Verification items for the finished model (mm, model axes). Face numbers are marked on the shaded views. A direction names the side the tool comes from. Coordinates: 2 decimals unless noted, no trailing zeros. Loops run counter-clockwise (first coordinate to the right, second up) from the corner with the lowest first, then second, coordinate; pieces in that order, holes last. Notation, with made-up numbers: M 10,-28.5 L 14,-28.5 A20 cw 14,-0.5 Z; hole C -13.5,82 d1. An arc over 180 degrees is marked long. Write item = value, one per line. Start each with the question number.
```python
from build123d import *

# Parameters (mm, degrees)
SKETCH1_W           = 40
SKETCH1_H           = 20
BOSS_EXTRUDE1_DEPTH = 37
BOSS_EXTRUDE2_DEPTH = 2
SKETCH3_R           = 6
BOSS_EXTRUDE3_DEPTH = 2
SKETCH4_R           = 2.75
BOSS_EXTRUDE4_DEPTH = 5
SKETCH5_W           = 7
SKETCH5_H           = 20
BOSS_EXTRUDE5_DEPTH = 3
SKETCH7_R           = 1.75
CUT_EXTRUDE3_DEPTH  = 44.0464865


with BuildPart() as part:
    # Sketch1 → Boss-Extrude1 (new body)
    with BuildSketch(Plane.XY):
        Rectangle(SKETCH1_W, SKETCH1_H)
    extrude(amount=BOSS_EXTRUDE1_DEPTH)

    # Sketch2 → Boss-Extrude2 (add)
    with BuildSketch(Plane.XY.offset(37)):
        with BuildLine():
            Line((-7.5, 10), (20, 10))
            Line((20, 10), (20, -10))
            Line((20, -10), (-7.5, -10))
            ThreePointArc((-7.5, -10), (-17.5, 0), (-7.5, 10))
        make_face()
    extrude(amount=BOSS_EXTRUDE2_DEPTH)

    # Sketch3 → Boss-Extrude3 (add)
    with BuildSketch(Plane.XY.offset(39)):
        with Locations((-7.5, 0)):
            Circle(SKETCH3_R)
    extrude(amount=BOSS_EXTRUDE3_DEPTH)

    # Sketch4 → Boss-Extrude4 (add)
    with BuildSketch(Plane.XY.offset(41)):
        with Locations((-7.5, 0)):
            Circle(SKETCH4_R)
    extrude(amount=BOSS_EXTRUDE4_DEPTH)

    # Sketch5 → Boss-Extrude5 (add)
    with BuildSketch(Plane.XY.offset(32)):
        with Locations((-23.5, 0)):
            Rectangle(SKETCH5_W, SKETCH5_H)
        with Locations((23.5, 0)):
            Rectangle(SKETCH5_W, SKETCH5_H)
    extrude(amount=-BOSS_EXTRUDE5_DEPTH)

    # Sketch7 → Cut-Extrude3 (cut, through all)
    with BuildSketch(Plane.XY.offset(32)):
        with Locations((-25.5, 5)):
            Circle(SKETCH7_R)
        with Locations((-25.5, -5)):
            Circle(SKETCH7_R)
        with Locations((25.5, -5)):
            Circle(SKETCH7_R)
        with Locations((25.5, 5)):
            Circle(SKETCH7_R)
    extrude(amount=-CUT_EXTRUDE3_DEPTH, mode=Mode.SUBTRACT)


solid = part.part
```
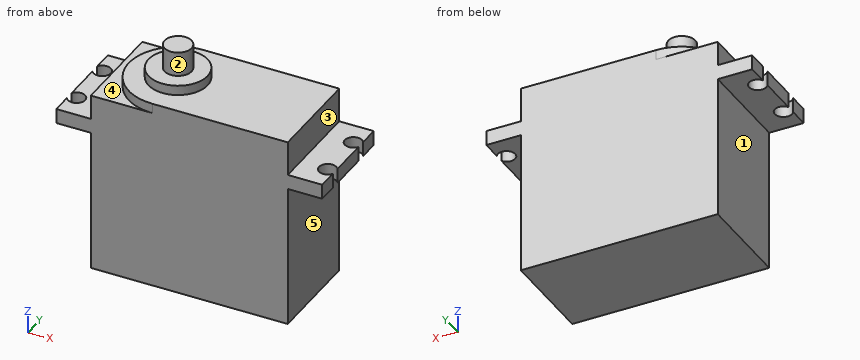
Q1. Scan lines: L1, parallel to Y at x = -25.5, z = 29.9; L2, parallel to Z at x = 3.5, y = 5.75; L3, parallel to X at y = 3.25, z = 27.5. Record each from-to range of solid material in increasing order. Write a range as [from, to].
Q2. Set-up check for the marked faces 1, 2, 3, 4 and 5: record each of +Z, -Z, +X, -X, +Y, -Y from which the full face is reachable in a straight line by a thin tool's end or side.
Q3. Sectioned sample at C-C on z = 25. Record the cut outline in (x, y), plus the area to 3 significant figures.
Q4. Sectioned sample at D-D on x = 14. Record the cut outline in (y, z).
Q5. Sectioned sample at A-A on x = 25.5. Record the cut outline in (y, z).
Q6. Gauge pin test, flat ends, axial feed: pin 1 (1 mm diameter, centred on y = -1, z = 19.5, fed in from +X); pin 2 (10 mm diameter, centred on x = 10.5, y = 0, fed in from +Z); pin 3 (4 mm diameter, centred on x = 25.5, y = 5, fed in from -Z). Record the tip position at first contact, or that the pin passes through.
Q7. Sectioned sample at B-B on y = 0. Record the cut outline in (x, z), plus the area to 3 significant figures.
Solutions:
q1.L1 = [-10, -6.75], [-3.25, 3.25], [6.75, 10]
q1.L2 = [0, 39]
q1.L3 = [-20, 20]
q2.face_1 = -Z, -X, +Y, -Y
q2.face_2 = +Z
q2.face_3 = +Z, +X, +Y, -Y
q2.face_4 = +Z, -X
q2.face_5 = -Z, +X, +Y, -Y
q3.outline = M -20,-10 L 20,-10 L 20,10 L -20,10 Z
q3.area = 800 mm²
q4.outline = M -10,0 L 10,0 L 10,39 L -10,39 Z
q5.outline = M -10,29 L -6.75,29 L -6.75,32 L -10,32 Z; M -3.25,29 L 3.25,29 L 3.25,32 L -3.25,32 Z; M 6.75,29 L 10,29 L 10,32 L 6.75,32 Z
q6.pin_1 = 20
q6.pin_2 = 39
q6.pin_3 = 29
q7.outline = M -27,29 L -20,29 L -20,0 L 20,0 L 20,29 L 27,29 L 27,32 L 20,32 L 20,39 L -1.5,39 L -1.5,41 L -4.75,41 L -4.75,46 L -10.25,46 L -10.25,41 L -13.5,41 L -13.5,39 L -17.5,39 L -17.5,37 L -20,37 L -20,32 L -27,32 Z
q7.area = 1,650 mm²
